Geometry: final body of the model. Coordinates: model frame, mm. A direction names the side the tool comes from. Coordinates: 2 decimals unless noted, no trailing zeros. Order: outer loops, then holes, each group sorted by start corner. A loop starts at its lowest first (then second) coordinate and runs counter-clockwise, first axis right, second up. Notation, with made-up numbers: (77, 63) -> (81, 63) arc R32 ccw to (81, 89) -> close; hole circle Ø10 at (47.25, -26.75). An arc over 180 degrees is marked (long way). Use CSV: the item, a comma, the result in double quotes. Start each with the question number.
from build123d import *

# Parameters (mm, degrees)
SKETCH1_W                                         = 46
SKETCH1_H                                         = 36
BOSS_EXTRUDE1_DEPTH                               = 8
F_3_0MM_DOWEL_HOLE1_D                             = 3
F_3_0MM_DOWEL_HOLE1_DEPTH                         = 8.5
F_3_0MM_DOWEL_HOLE1_TIP                           = 0.901290929
F_4_0MM_DOWEL_HOLE1_D                             = 4
F_4_0MM_DOWEL_HOLE1_DEPTH                         = 7.5
F_4_0MM_DOWEL_HOLE1_TIP                           = 1.201721238
FILLET2_R                                         = 8
SKETCH16_W                                        = 5
SKETCH16_H                                        = 5
CUT_EXTRUDE1_DEPTH                                = 4.5
CSK_FOR_M2_5_FLAT_HEAD_MACHINE_SCREW1_D           = 2.5
CSK_FOR_M2_5_FLAT_HEAD_MACHINE_SCREW1_DEPTH       = 9.5
CSK_FOR_M2_5_FLAT_HEAD_MACHINE_SCREW1_CSINK_D     = 5.5
CSK_FOR_M2_5_FLAT_HEAD_MACHINE_SCREW1_CSINK_ANGLE = 90
CSK_FOR_M2_5_FLAT_HEAD_MACHINE_SCREW1_TIP         = 0.751075774
HOLE1_D                                           = 10
HOLE1_CBORE_D                                     = 12
HOLE1_CBORE_DEPTH                                 = 3.3
F_3_0_3_DIAMETER_HOLE1_D                          = 3
FILLET3_R                                         = 1
CUT_EXTRUDE2_DEPTH                                = 4


with BuildPart() as part:
    # Sketch1 → Boss-Extrude1 (new body)
    with BuildSketch(Plane.XY.offset(4.5)):
        Rectangle(SKETCH1_W, SKETCH1_H)
    extrude(amount=-BOSS_EXTRUDE1_DEPTH)

    # Ø3.0mm Dowel Hole1
    with Locations(Plane(origin=(0, -18, 0), x_dir=(-1, 0, 0), z_dir=(0, -1, 0))):
        with Locations((0, -0.5)):
            Hole(F_3_0MM_DOWEL_HOLE1_D / 2, depth=F_3_0MM_DOWEL_HOLE1_DEPTH)
            with Locations((0, 0, -(F_3_0MM_DOWEL_HOLE1_DEPTH + F_3_0MM_DOWEL_HOLE1_TIP / 2))):  # 118° drill point
                Cone(0, F_3_0MM_DOWEL_HOLE1_D / 2, F_3_0MM_DOWEL_HOLE1_TIP, mode=Mode.SUBTRACT)

    # Ø4.0mm Dowel Hole1
    with Locations(Plane(origin=(0, -18, 0), x_dir=(-1, 0, 0), z_dir=(0, -1, 0))):
        with Locations((19, -0.5), (-19, -0.5)):
            Hole(F_4_0MM_DOWEL_HOLE1_D / 2, depth=F_4_0MM_DOWEL_HOLE1_DEPTH)
            with Locations((0, 0, -(F_4_0MM_DOWEL_HOLE1_DEPTH + F_4_0MM_DOWEL_HOLE1_TIP / 2))):  # 118° drill point
                Cone(0, F_4_0MM_DOWEL_HOLE1_D / 2, F_4_0MM_DOWEL_HOLE1_TIP, mode=Mode.SUBTRACT)

    # Fillet2
    fillet2_edges = [part.edges().sort_by_distance(p)[0] for p in [
        (-23, 18, 0.5),
        (23, 18, 0.5),
    ]]
    fillet(fillet2_edges, radius=FILLET2_R)

    # Sketch16 → Cut-Extrude1 (cut)
    with BuildSketch(Plane(origin=(0, 0, -3.5), x_dir=(-1, 0, 0), z_dir=(0, 0, -1))):
        with Locations((5, -2)):
            Rectangle(SKETCH16_W, SKETCH16_H)
    extrude(amount=-CUT_EXTRUDE1_DEPTH, mode=Mode.SUBTRACT)

    # CSK for M2.5 Flat Head Machine Screw1
    with Locations(Plane(origin=(-5, -2, 4.5), x_dir=(1, 0, 0), z_dir=(0, 0, 1))):
        with Locations((0, 0)):
            CounterSinkHole(CSK_FOR_M2_5_FLAT_HEAD_MACHINE_SCREW1_D / 2, CSK_FOR_M2_5_FLAT_HEAD_MACHINE_SCREW1_CSINK_D / 2, depth=CSK_FOR_M2_5_FLAT_HEAD_MACHINE_SCREW1_DEPTH, counter_sink_angle=CSK_FOR_M2_5_FLAT_HEAD_MACHINE_SCREW1_CSINK_ANGLE)
            with Locations((0, 0, -(CSK_FOR_M2_5_FLAT_HEAD_MACHINE_SCREW1_DEPTH + CSK_FOR_M2_5_FLAT_HEAD_MACHINE_SCREW1_TIP / 2))):  # 118° drill point
                Cone(0, CSK_FOR_M2_5_FLAT_HEAD_MACHINE_SCREW1_D / 2, CSK_FOR_M2_5_FLAT_HEAD_MACHINE_SCREW1_TIP, mode=Mode.SUBTRACT)

    # Hole1 (through all)
    with Locations(Plane.XY.offset(4.5)):
        with Locations((-0.625, 5.577722283)):
            CounterBoreHole(HOLE1_D / 2, HOLE1_CBORE_D / 2, HOLE1_CBORE_DEPTH)

    # Ø3.0 (3) Diameter Hole1 (through all)
    with Locations(Plane(origin=(0, 0, -3.5), x_dir=(-1, 0, 0), z_dir=(0, 0, -1))):
        with Locations((-8.703529058, 11.40683419), (10.337423522, 10.741909474), (0.241105536, -5.415576814)):
            Hole(F_3_0_3_DIAMETER_HOLE1_D / 2)

    # Fillet3
    fillet3_edges = [part.edges().sort_by_distance(p)[0] for p in [
        (-7.5, 0.5, -1.25),
        (-7.5, -4.5, -1.25),
        (-2.5, -4.5, -1.25),
        (-2.5, 0.5, -1.25),
    ]]
    fillet(fillet3_edges, radius=FILLET3_R)

    # Sketch20 → Cut-Extrude2 (cut)
    with BuildSketch(Plane(origin=(0, 0, -3.5), x_dir=(-1, 0, 0), z_dir=(0, 0, -1))):
        Polygon((14.378875406, 10.741909474), (12.358149464, 14.241909474), (8.316697579, 14.241909474), (6.295971637, 10.741909474), (8.316697579, 7.241909474), (12.358149464, 7.241909474), align=None)
    extrude(amount=-CUT_EXTRUDE2_DEPTH, mode=Mode.SUBTRACT)


solid = part.part
(1) Section C-C (x = -5). Return loops of the section in (y, z), then the cut area to 3 significant figures.
(2) Section D-D (z = 0). State how many separate pieces and enclosed holes the cut face has, then the cut area to 3 significant figures.
(3) Mould query, pull axis Y, two halves, no side actions, for faces 1 (the face through (23, -4, 1)), 2 (the face through (-7.5, -2, -1)), 3 (the face through (20.594, 15.719, 0.444)). Classes: pulls with the +Y half, pulls with the -Y half, needs draft (parallel to the pull), parting line crosses it, or undercut.
(4) Line query: line 1 (X direction, y = -2, z = 1.85); line 2 (Y direction, x = -11.5, z = -2.5); line 3 (X direction, y = -11, z = 0). Output: solid intervals per line, ascending. Write a range as from..to.
(5) Access query for faces 4 (the face through (-2.785, -4.199, -1.219)), 5 (the face through (-4, 10, 1.2)), 6 (the face through (-0.3, -3.7, 4.5)), 7 (the face through (0, -14, 2)), 8 (the face through (0.026, 10.535, -1.183)). Directions: +Z, -Z, +X, -X, +Y, -Y. A direction counts if a zero-diameter tool reaches every point of the face in a straight line with its end or side. Return the directions, or none.
(6) Section B-B (x = 9). Return loops of the section in (y, z).
(7) First-contact query: pin 1 (3.5 mm diameter, centred on x = -1.5, y = 8, fed in from +Z); pin 2 (2.5 mm diameter, centred on x = 0, z = 0.5, fed in from -Y); pin 3 (7.5 mm diameter, centred on x = -9, y = 10.5, fed in from -Z); pin 4 (1.5 mm diameter, centred on x = -4.5, y = -2.5, fed in from -Z). Flat tips, straight axial feed; report the tip coordinate or a pass-through.
(8) Section A-A (y = -2). Return loops of the section in (x, z), then the cut area to 4 significant figures.
Check sheet entries:
1,outline,"(-18, -3.5) -> (-4.5, -3.5) -> (-4.5, 1) -> (-3.25, 1) -> (-3.25, 3) -> (-4.75, 4.5) -> (-18, 4.5) -> close; (-0.75, 1) -> (0.5, 1) -> (0.5, -3.5) -> (3.16, -3.5) -> (3.16, 1.2) -> (1.47, 1.2) -> (1.47, 4.5) -> (0.75, 4.5) -> (-0.75, 3) -> close; (8, -3.5) -> (18, -3.5) -> (18, 4.5) -> (9.68, 4.5) -> (9.68, 1.2) -> (8, 1.2) -> close"
1,area,"205 mm^2"
2,separate pieces,"1"
2,enclosed holes,"5"
2,area,"1,380 mm^2"
3,face 1,"needs draft"
3,face 2,"undercut"
3,face 3,"pulls with the +Y half"
4,line 1,"x = -23..-6.25, -3.75..23"
4,line 2,"y = -18..7.24, 14.24..18"
4,line 3,"x = -23..-20.94, -17.06..-1.41, 1.41..17.06, 20.94..23"
5,face 4,"-Z"
5,face 5,"+Z"
5,face 6,"+Z, +X, -X, +Y, -Y"
5,face 7,"-Y"
5,face 8,"+Z, -Z"
6,outline,"(-18, -3.5) -> (9.94, -3.5) -> (9.94, 4.5) -> (-18, 4.5) -> close; (12.88, -3.5) -> (18, -3.5) -> (18, 4.5) -> (12.88, 4.5) -> close"
7,pin 1,"passes through"
7,pin 2,"stops at y = -9.35"
7,pin 3,"stops at z = -3.5"
7,pin 4,"stops at z = 1"
8,outline,"(-23, -3.5) -> (-7.5, -3.5) -> (-7.5, 1) -> (-6.25, 1) -> (-6.25, 3) -> (-7.75, 4.5) -> (-23, 4.5) -> close; (-3.75, 1) -> (-2.5, 1) -> (-2.5, -3.5) -> (23, -3.5) -> (23, 4.5) -> (-2.25, 4.5) -> (-3.75, 3) -> close"
8,area,"334.5 mm^2"
